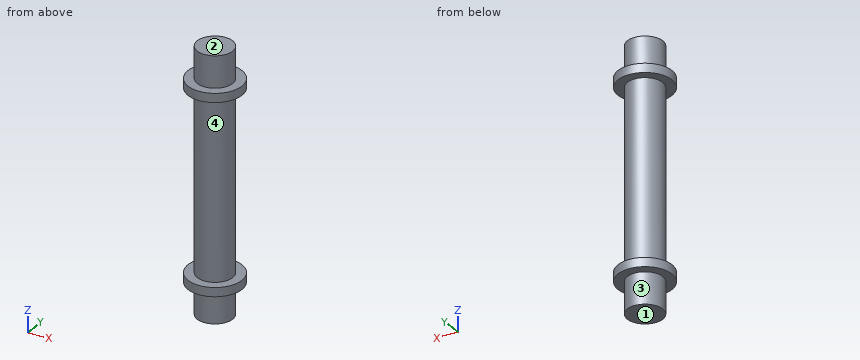
```python
from build123d import *

# Parameters (mm, degrees)
SKETCH1_R           = 3.95
BOSS_EXTRUDE1_DEPTH = 58
SKETCH2_R           = 6
BOSS_EXTRUDE2_DEPTH = 2
BOSS_EXTRUDE3_START = -2
SKETCH3_R           = 6
BOSS_EXTRUDE3_DEPTH = 2


with BuildPart() as part:
    # Sketch1 → Boss-Extrude1 (new body)
    with BuildSketch(Plane.XY):
        with Locations(Location((0, 0, 0), (0, 0, 180))):
            Circle(SKETCH1_R)
    extrude(amount=BOSS_EXTRUDE1_DEPTH)

    # Sketch2 → Boss-Extrude2 (add)
    with BuildSketch(Plane.XY.offset(51)):
        Circle(SKETCH2_R)
    extrude(amount=-BOSS_EXTRUDE2_DEPTH)

    # Sketch3 → Boss-Extrude3 (add)
    with BuildSketch(Plane(origin=(0, 0, 7), x_dir=(-1, 0, 0), z_dir=(0, 0, -1)).offset(BOSS_EXTRUDE3_START)):
        with Locations(Location((0, 0, 0), (0, 0, 180))):
            Circle(SKETCH3_R)
    extrude(amount=BOSS_EXTRUDE3_DEPTH)


solid = part.part
```
Can you work these out from the model? Positions are in its coordinate system, mm. Face numbers are marked on the shaded views. Coordinates: 2 decimals unless noted, no trailing zeros. Loops run counter-clockwise (first coordinate to the right, second up) from the corner with the lowest first, then second, coordinate; pieces in that order, holes last. Notation, with made-up numbers: (40.25, -21.5) - (58.25, -21.5) arc R29 cw to (58.25, 14.5) - close; hole circle Ø2 at (80.25, -7.5). An arc over 180 degrees is marked (long way). Use a Markdown table: item, result.
Item 1: Will these pins go through, and if not, where does the flat tip stop? pin 1 (6 mm diameter, centred on y = -1, z = 33, fed in from +X); pin 2 (6 mm diameter, centred on y = -4, z = 45, fed in from +X); pin 3 (1.5 mm diameter, centred on x = -3.5, z = 52, fed in from -Y).
Numbers:
| item | result |
|---|---|
| pin 1 | stops at x = 3.95 |
| pin 2 | stops at x = 3.82 |
| pin 3 | stops at y = -2.84 |
Item 2: If I drill on probe 1 along Z at (x, y) = (-4.25, 3.25); probe 2 along X at (y, z) = (1.75, 11.5); probe 3 along Y at (x, z) = (-3.5, 32), over which ranges is the centre line in solid material (lowest first)? Write a range as from..to.
Numbers:
| item | result |
|---|---|
| probe 1 | z = 7..9, 49..51 |
| probe 2 | x = -3.54..3.54 |
| probe 3 | y = -1.83..1.83 |
Item 3: I want a section at D-D on z = 17. Please give me the cut outline in (x, y).
Numbers:
| item | result |
|---|---|
| outline | circle Ø7.9 at (0, 0) |
Item 4: I want a section at B-B on x = 0. Please give me the cut outline in (y, z), and give its area (3 significant figures).
Numbers:
| item | result |
|---|---|
| outline | (-6, 7) - (-3.95, 7) - (-3.95, 0) - (3.95, 0) - (3.95, 7) - (6, 7) - (6, 9) - (3.95, 9) - (3.95, 49) - (6, 49) - (6, 51) - (3.95, 51) - (3.95, 58) - (-3.95, 58) - (-3.95, 51) - (-6, 51) - (-6, 49) - (-3.95, 49) - (-3.95, 9) - (-6, 9) - close |
| area | 475 mm2 |
Item 5: We'd pull the mould along Z, two halves only. Please class the marked faces 1, 2, 3 and 4: released by +Z, released by -Z, zero draft, split by the parting line, or undercut.
Numbers:
| item | result |
|---|---|
| face 1 | released by -Z |
| face 2 | released by +Z |
| face 3 | zero draft |
| face 4 | undercut |
Item 6: I want a section at A-A on y = 4.75. Please give me the cut outline in (x, z), and give its area (3 significant figures).
Numbers:
| item | result |
|---|---|
| outline | (-3.67, 7) - (3.67, 7) - (3.67, 9) - (-3.67, 9) - close; (-3.67, 49) - (3.67, 49) - (3.67, 51) - (-3.67, 51) - close |
| area | 29.3 mm2 |
